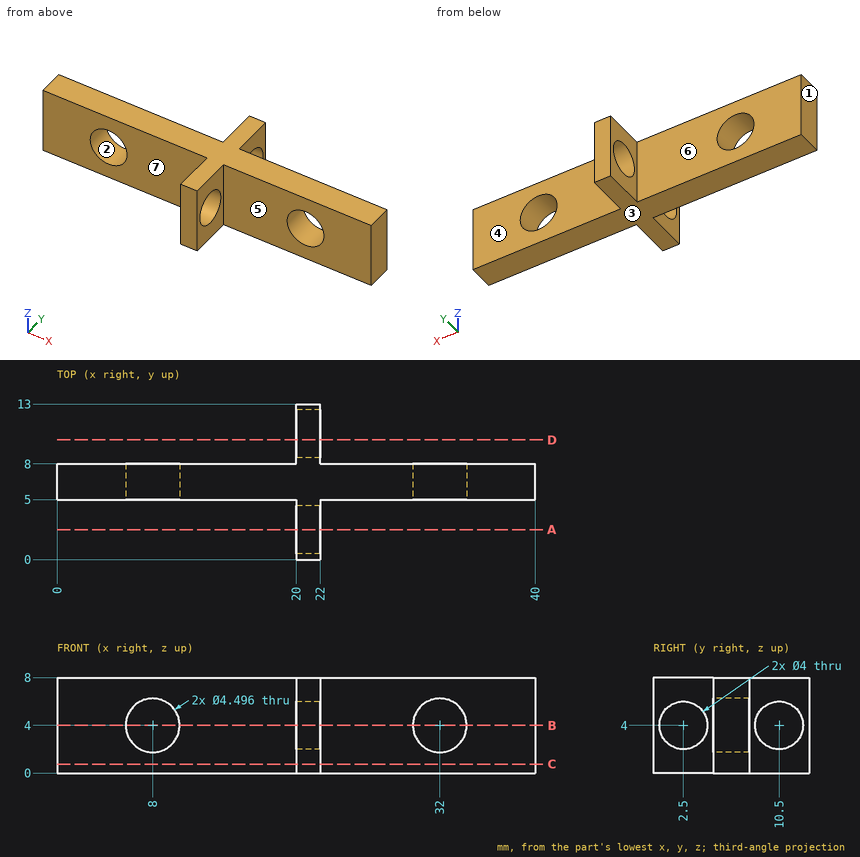
Geometry: see drawing. Coordinates: mm, zero at the bounding-box minimum. A direction names the side the tool comes from. Coordinates: 2 decimals unless noted, no trailing zeros. Order: outer loops, then holes, each group sorted by start corner. A loop starts at its lowest first (then second) coordinate and runs counter-clockwise, first axis right, second up. Notation, with made-up numbers: (6, 9) -> (42, 9) arc R18 ccw to (42, 13) -> close; hole circle Ø6 at (-2, 14). An arc over 180 degrees is marked (long way). Write each question's results on one line, items separated by ' | '. Start each with the question number.
1) Material intervals for line 1 along Y through (x, z) = (20.75, 4); line 2 along X through (y, z) = (6.8, 4); line 3 along Y through (x, z) = (23, 5.5), sorted ascending.
2) Mould query, pull axis X, two halves, no side actions, for the marked faces 1, 2 and 3. Classes: released by +X, released by -X, zero draft, split by the parting line, or undercut.
3) Cut plane B-B, the plane z = 4. Output: boundary loops of the cut face in (x, y).
4) Cut plane D-D, the plane y = 10. Output: boundary loops of the cut face in (x, z).
5) Set-up query: the marked faces 4, 5, 6 and 7. Return all of +Z, -Z, +X, -X, +Y, -Y with unobstructed straight access to the full face (end or side cutting, diameter ignored); none if empty.
6) First-contact query: pin 1 (1.5 mm diameter, centred on y = 3.5, z = 2, fed in from +X); pin 2 (3 mm diameter, centred on x = 15, z = 7, fed in from -Y); pin 3 (2 mm diameter, centred on x = 34.5, z = 1, fed in from +Y). Flat tips, straight axial feed; report the tip coordinate or a pass-through.
7) Cut plane C-C, the plane z = 0.75. Output: boundary loops of the cut face in (x, y).
8) Cut plane A-A, the plane y = 2.5. Output: boundary loops of the cut face in (x, z).
Checks:
1) line 1: 0 to 0.5, 4.5 to 8.5, 12.5 to 13 | line 2: 0 to 5.75, 10.25 to 29.75, 34.25 to 40 | line 3: 5 to 8
2) face 1: released by -X | face 2: undercut | face 3: zero draft
3) outline: (0, 5) -> (5.75, 5) -> (5.75, 8) -> (0, 8) -> close; (10.25, 5) -> (20, 5) -> (20, 4.5) -> (22, 4.5) -> (22, 5) -> (29.75, 5) -> (29.75, 8) -> (22, 8) -> (22, 8.5) -> (20, 8.5) -> (20, 8) -> (10.25, 8) -> close; (20, 0) -> (22, 0) -> (22, 0.5) -> (20, 0.5) -> close; (20, 12.5) -> (22, 12.5) -> (22, 13) -> (20, 13) -> close; (34.25, 5) -> (40, 5) -> (40, 8) -> (34.25, 8) -> close
4) outline: (20, 0) -> (22, 0) -> (22, 2.06) -> (20, 2.06) -> close; (20, 5.94) -> (22, 5.94) -> (22, 8) -> (20, 8) -> close
5) face 4: +Z, -Z, +X, +Y | face 5: +Z, -Z, +X, -Y | face 6: +Z, -Z, -X, +Y | face 7: +Z, -Z, -X, -Y
6) pin 1: x = 22 | pin 2: y = 5 | pin 3: y = 8
7) outline: (0, 5) -> (20, 5) -> (20, 0) -> (22, 0) -> (22, 5) -> (40, 5) -> (40, 8) -> (22, 8) -> (22, 13) -> (20, 13) -> (20, 8) -> (0, 8) -> close
8) outline: (20, 0) -> (22, 0) -> (22, 2) -> (20, 2) -> close; (20, 6) -> (22, 6) -> (22, 8) -> (20, 8) -> close
